```python
from build123d import *

# Parameters (mm, degrees)
SKETCH1_R           = 18
BOSS_EXTRUDE1_DEPTH = 8.8
SKETCH2_W           = 7.2
SKETCH2_H           = 10.2
CUT_EXTRUDE1_DEPTH  = 2.2


with BuildPart() as part:
    # Sketch1 → Boss-Extrude1 (new body)
    with BuildSketch(Plane(origin=(0, 0, 0), x_dir=(1, 0, 0), z_dir=(0, 1, 0))):
        with Locations(Location((0, 0, 0), (0, 0, 270))):
            Circle(SKETCH1_R)
    extrude(amount=BOSS_EXTRUDE1_DEPTH)

    # Sketch2 → Cut-Extrude1 (cut)
    with BuildSketch(Plane(origin=(0, 8.8, 0), x_dir=(1, 0, 0), z_dir=(0, 1, 0))):
        with Locations((-9.6, 0)):
            Rectangle(SKETCH2_W, SKETCH2_H)
        with Locations((9.6, 0)):
            Rectangle(SKETCH2_W, SKETCH2_H)
    extrude(amount=-CUT_EXTRUDE1_DEPTH, mode=Mode.SUBTRACT)


solid = part.part
```
The listing builds one solid part. Answer for the finished solid, in the listing's coordinates (mm). A direction names the side the tool comes from. Coordinates: 2 decimals unless noted, no trailing zeros. Write each loop counter-clockwise with the first axis right and the second up, starting at its lowest first coordinate (ties: lowest second). Pieces come first, ordered by that corner, then holes. Notation, with made-up numbers: (-36, 74) -> (22, 74) arc R20 cw to (22, 100) -> close; hole circle Ø10 at (-7.75, -38.75). An arc over 180 degrees is marked (long way). Write each question's results on one line, items separated by ' | '. Start each with the question number.
1) A tool of negligible diameter and unlimited length cuts with its end or side. For faces 1 (the flat face through (0, 8.8, 0)), 2 (the flat face through (-10, 8, -5.1)), from which of +Z, -Z, +X, -X, +Y, -Y can it reach the whole face along a straight path? Write none if from no direction.
2) Straight lines are drawn through the part: probe 1 along X at (y, z) = (7, 5); probe 2 along Y at (x, z) = (12, -4); probe 3 along X at (y, z) = (3.5, 6). For each, find the intervals that lie inside material, in ascending order.
3) A cutting plane is placed at D-D (x = 7). Determine the outline of the cut face in (y, z).
4) A cutting plane is placed at A-A (z = 0). Determine the outline of the cut face in (x, y).
5) A cutting plane is placed at B-B (x = 12). Determine the outline of the cut face in (y, z), then the cut area to 3 significant figures.
6) A cutting plane is placed at C-C (y = 4.25). Determine the outline of the cut face in (x, z).
7) For a pull along X with two mould halves and no side action, classify faces 3 (the flat face through (0, 0, 0)), 4 (the cylindrical face through (5.407, 4.338, 17.169)), 5 (the flat face through (-13.2, 8, 0)) as +X half, -X half, draft (parallel to the pull), parting line (faces both ways), or undercut.
8) Flat-ended cylindrical pins translate along their axes: pin 1 Ø2 at (y, z) = (4, -4.5) entering from -X; pin 2 Ø4 at (y, z) = (1, -8.5) entering from -X; pin 3 Ø2.5 at (y, z) = (7.5, -0.5) entering from -X. Find the tip coordinate at first contact, or state that the pin passes through.
Values follow:
1) face 1: +Z, -Z, +X, -X, +Y | face 2: +Y
2) probe 1: -17.29 to -13.2, -6 to 6, 13.2 to 17.29 | probe 2: 0 to 6.6 | probe 3: -16.97 to 16.97
3) outline: (0, -16.58) -> (8.8, -16.58) -> (8.8, -5.1) -> (6.6, -5.1) -> (6.6, 5.1) -> (8.8, 5.1) -> (8.8, 16.58) -> (0, 16.58) -> close
4) outline: (-18, 0) -> (18, 0) -> (18, 8.8) -> (13.2, 8.8) -> (13.2, 6.6) -> (6, 6.6) -> (6, 8.8) -> (-6, 8.8) -> (-6, 6.6) -> (-13.2, 6.6) -> (-13.2, 8.8) -> (-18, 8.8) -> close
5) outline: (0, -13.42) -> (8.8, -13.42) -> (8.8, -5.1) -> (6.6, -5.1) -> (6.6, 5.1) -> (8.8, 5.1) -> (8.8, 13.42) -> (0, 13.42) -> close | area: 214 mm²
6) outline: circle Ø36 at (0, 0)
7) face 3: draft | face 4: parting line | face 5: undercut
8) pin 1: x = -17.66 | pin 2: x = -16.79 | pin 3: x = -18
